from build123d import *

# Parameters (mm, degrees)
SKETCH_R        = 1.7
PAD_DEPTH       = 24
SKETCH001_W     = 35
SKETCH001_H     = 16
POCKET_DEPTH    = 57
SKETCH002_W     = 20
SKETCH002_H     = 8
POCKET001_DEPTH = 5
SKETCH003_W     = 11
SKETCH003_H     = 20
POCKET002_DEPTH = 40.001
SKETCH004_W     = 20
SKETCH004_H     = 15
SKETCH004_R     = 1.7
PAD001_DEPTH    = 6
SKETCH005_W     = 12
SKETCH005_H     = 2.2
POCKET003_DEPTH = 40.001
SKETCH006_W     = 12
SKETCH006_H     = 12
PAD002_DEPTH    = 8.5
SKETCH007_R     = 2.7
POCKET004_DEPTH = 30.001
SKETCH008_W     = 12
SKETCH008_H     = 8
POCKET005_DEPTH = 6
POCKET006_DEPTH = 10
SKETCH010_W     = 7.6
SKETCH010_H     = 2.2
POCKET007_DEPTH = 2
POCKET008_DEPTH = 3.001
POCKET009_DEPTH = 5


with BuildPart() as part:
    # Sketch → Pad (new body)
    with BuildSketch(Plane.XY):
        with BuildLine():
            Line((3, 41), (20, 41))
            Line((20, 41), (20, 52))
            Line((20, 52), (40, 52))
            Line((40, 52), (40, 41))
            Line((40, 41), (57, 41))
            ThreePointArc((60, 38), (59.12132, 40.12132), (57, 41))
            Line((60, 38), (60, 3))
            ThreePointArc((57, 0), (59.12132, 0.87868), (60, 3))
            Line((57, 0), (3, 0))
            ThreePointArc((0, 3), (0.87868, 0.87868), (3, 0))
            Line((0, 3), (0, 38))
            ThreePointArc((3, 41), (0.87868, 40.12132), (0, 38))
        make_face()
        with Locations((30, 45)):
            Circle(SKETCH_R, mode=Mode.SUBTRACT)
        with BuildLine():
            Line((7, 4), (53, 4))
            ThreePointArc((53, 4), (55.12132, 4.87868), (56, 7))
            Line((56, 7), (56, 34))
            ThreePointArc((56, 34), (55.12132, 36.12132), (53, 37))
            Line((53, 37), (7, 37))
            ThreePointArc((7, 37), (4.87868, 36.12132), (4, 34))
            Line((4, 34), (4, 7))
            ThreePointArc((4, 7), (4.87868, 4.87868), (7, 4))
        make_face(mode=Mode.SUBTRACT)
    extrude(amount=PAD_DEPTH)

    # Sketch001 → Pocket (cut)
    with BuildSketch(Plane(origin=(0, 0, 0), x_dir=(0, -1, 0), z_dir=(-1, 0, 0))):
        with Locations((-20.5, 12)):
            Rectangle(SKETCH001_W, SKETCH001_H)
    extrude(amount=-POCKET_DEPTH, mode=Mode.SUBTRACT)

    # Sketch002 → Pocket001 (cut)
    with BuildSketch(Plane.YZ.offset(60)):
        with Locations((21, 8)):
            Rectangle(SKETCH002_W, SKETCH002_H)
    extrude(amount=-POCKET001_DEPTH, mode=Mode.SUBTRACT)

    # Sketch003 → Pocket002 (cut, through all)
    with BuildSketch(Plane(origin=(20, 0, 0), x_dir=(0, -1, 0), z_dir=(-1, 0, 0))):
        with Locations((-46.5, 14)):
            Rectangle(SKETCH003_W, SKETCH003_H)
    extrude(amount=-POCKET002_DEPTH, mode=Mode.SUBTRACT)

    # Sketch004 → Pad001 (new body)
    with BuildSketch(Plane(origin=(0, 0, 0), x_dir=(1, 0, 0), z_dir=(0, 0, -1))):
        with Locations((30, -44.5)):
            Rectangle(SKETCH004_W, SKETCH004_H)
        with Locations((30, -45)):
            Circle(SKETCH004_R, mode=Mode.SUBTRACT)
    extrude(amount=PAD001_DEPTH)

    # Sketch005 → Pocket003 (cut, through all)
    with BuildSketch(Plane.YZ.offset(40)):
        with Locations((43, -1.1)):
            Rectangle(SKETCH005_W, SKETCH005_H)
    extrude(amount=-POCKET003_DEPTH, mode=Mode.SUBTRACT)

    # Sketch006 → Pad002 (new body)
    with BuildSketch(Plane.YZ.offset(60)):
        with Locations((21, 18)):
            Rectangle(SKETCH006_W, SKETCH006_H)
    extrude(amount=PAD002_DEPTH)

    # Sketch007 → Pocket004 (cut, through all)
    with BuildSketch(Plane.XY.offset(24)):
        with Locations((62.7, 21)):
            Circle(SKETCH007_R)
    extrude(amount=-POCKET004_DEPTH, mode=Mode.SUBTRACT)

    # Sketch008 → Pocket005 (cut)
    with BuildSketch(Plane.YZ.offset(68.5)):
        with Locations((21, 18)):
            Rectangle(SKETCH008_W, SKETCH008_H)
    extrude(amount=-POCKET005_DEPTH, mode=Mode.SUBTRACT)

    # Sketch009 → Pocket006 (cut)
    with BuildSketch(Plane.YZ.offset(62.5)):
        with BuildLine():
            ThreePointArc((17.2, 19.200001), (16.5, 19.900001), (15.8, 19.200001))
            Line((15.8, 19.200001), (15.8, 17))
            ThreePointArc((15.8, 17), (16.5, 16.3), (17.2, 17.000001))
            Line((17.2, 19.200001), (17.2, 17.000001))
        make_face()
        with BuildLine():
            ThreePointArc((26.2, 19.2), (25.5, 19.900001), (24.8, 19.200001))
            Line((24.8, 19.200001), (24.8, 17.000001))
            ThreePointArc((24.8, 17.000001), (25.5, 16.300001), (26.2, 17))
            Line((26.2, 19.2), (26.2, 17))
        make_face()
    extrude(amount=-POCKET006_DEPTH, mode=Mode.SUBTRACT)

    # Sketch010 → Pocket007 (cut)
    with BuildSketch(Plane(origin=(57, 0, 0), x_dir=(0, -1, 0), z_dir=(-1, 0, 0))):
        with Locations((-21, 18.100001)):
            Rectangle(SKETCH010_W, SKETCH010_H)
    extrude(amount=-POCKET007_DEPTH, mode=Mode.SUBTRACT)

    # Sketch011 → Pocket008 (cut, through all)
    with BuildSketch(Plane(origin=(0, 3, 0), x_dir=(-1, 0, 0), z_dir=(0, 1, 0))):
        with BuildLine():
            ThreePointArc((-1.4, 12.999991), (-2, 13.6), (-2.6, 12.999991))
            Line((-2.6, 12.999991), (-2.6, 10.799995))
            ThreePointArc((-2.6, 10.799995), (-2, 10.2), (-1.4, 10.799994))
            Line((-1.4, 12.999991), (-1.4, 10.799994))
        make_face()
    extrude(amount=-POCKET008_DEPTH, mode=Mode.SUBTRACT)

    # Sketch012 → Pocket009 (cut)
    with BuildSketch(Plane.XZ.offset(-38)):
        with BuildLine():
            ThreePointArc((3.2, 13), (2.6, 13.600002), (2, 13))
            Line((2, 13), (2, 10.800003))
            ThreePointArc((2, 10.800003), (2.6, 10.200002), (3.2, 10.800003))
            Line((3.2, 13), (3.2, 10.800003))
        make_face()
    extrude(amount=-POCKET009_DEPTH, mode=Mode.SUBTRACT)


solid = part.part
For this review, take the finished solid that the model builds, in its own axes (mm). A direction names the side the tool comes from. Round coordinates to 2 decimals unless told otherwise and drop trailing zeros. Write each loop counter-clockwise with the first axis right and the second up, starting at its lowest first coordinate (ties: lowest second). Pieces come first, ordered by that corner, then holes. Notation, with made-up numbers: M -12.5,1 L 9.5,1 A21 cw 9.5,24 Z; hole C 35,77 d7. An arc over 180 degrees is marked long. Write item = value, one per line. Start each with the question number.
(1) We need section C-C (x = 30). Give the number of separate pieces and of enclosed holes in the cut face, then the cut area to 3 significant figures.
(2) We need section A-A (y = 32). Give the boundary of the cut face in (x, z).
(3) We need section B-B (z = 21). Give the boundary of the cut face in (x, y).
(4) For faces 5 (the face through (4.9, 36.14, 21.97)), 6 (the face through (60, 15.8, 18)), 7 (the face through (28, 3, 12)), 8 (the face through (62.5, 17.4, 18.1)), list the 3-axis set-ups (+Z, -Z, +X, -X, +Y, -Y) from which the entire face can be reached by the end or side of a thin tool; tool diameter is ignored.
(5) For line 1 along Z through (x, y) = (37.5, 37.5); line 2 along Y through (x, z) = (41, 14); line 3 along X through (y, z) = (30, 2), list the stretches that pass through material, from the lowest coordinate up.
(6) Clearance check with flat-ended pins moving along their axes: pin 1 Ø2.5 at (x, z) = (60.5, 17.5) entering from -Y; pin 2 Ø3 at (x, y) = (65, 19.5) entering from -Z; pin 3 Ø10 at (y, z) = (6, 14.5) entering from +X. State where each tip first meets the part, or that it passes through.
(7) The part is to be moulded in two halves that separate along Y. For faces 1 (the face through (0.86, 0.9, 11.83)), 2 (the face through (59.14, 40.1, 11.83)), 3 (the face through (68.5, 21, 13)), 4 (the face through (56, 20, 2)), say which applies: +Y half, -Y half, draft (parallel to the pull), parting line (faces both ways), or undercut.
Results found:
q1.separate_pieces = 4
q1.enclosed_holes = 0
q1.area = 241 mm²
q2.outline = M 0,0 L 4,0 L 4,4 L 0,4 Z; M 0,20 L 4,20 L 4,24 L 0,24 Z; M 56,0 L 60,0 L 60,24 L 56,24 L 56,20 L 57,20 L 57,4 L 56,4 Z
q3.outline = M 0,3 A3 ccw 3,0 L 57,0 A3 ccw 60,3 L 60,15 L 62.5,15 L 62.5,18.31 A2.7 cw 62.5,23.69 L 62.5,27 L 60,27 L 60,38 A3 ccw 57,41 L 3,41 A3 ccw 0,38 Z; hole M 4,7 A3 ccw 7,4 L 53,4 A3 ccw 56,7 L 56,34 A3 ccw 53,37 L 7,37 A3 ccw 4,34 Z
q4.face_5 = +Z, -Z
q4.face_6 = +X, -X
q4.face_7 = -X
q4.face_8 = +X, +Y, -Y
q5.line_1 = -6 to -2.2, 0 to 4, 20 to 24
q5.line_2 = 0 to 3, 38 to 41
q5.line_3 = 0 to 4, 56 to 60
q6.pin_1 = 1.02
q6.pin_2 = 12
q6.pin_3 = 60
q7.face_1 = -Y half
q7.face_2 = +Y half
q7.face_3 = draft
q7.face_4 = undercut
